Part model, mm, in its own coordinate system. A direction names the side the tool comes from. Give positions to 0.01 mm unless a question says otherwise; leave off trailing zeros. Write each loop counter-clockwise with the first axis right and the second up, starting at its lowest first coordinate (ties: lowest second). Pieces come first, ordered by that corner, then holes. Notation, with made-up numbers: (-12.5, 3) - (17.5, 3) arc R24 cw to (17.5, 34) - close; hole circle Ø9 at (16, 22.5). An arc over 180 degrees is marked (long way). Answer in a Markdown table with one row per item. Add a question column.
1. Probe line 1 along X through (y, z) = (-5.5, 216); line 2 along Z through (x, y) = (-749.3, -17.5); line 3 along Z through (x, y) = (-891.5, -16). List the from-to ranges inside material, lowest first.
2. Band-saw the part on A-A on y = -15.25. State how many separate pieces and enclosed holes the cut face has, plus the area to 3 significant figures.
3. Which spindle directions (+Z, -Z, +X, -X, +Y, -Y) get a long thin tool onto all of the face, cutting with end or side? Do faces 1 (the flat face through (-1172, -13, 152.4)), 2 (the flat face through (-1473.2, -13, 283)), 3 (the flat face through (-1161, -13, 410.362)). Say none if no direction does.
4. Drop flat-ended pins along their axis: pin 1 Ø3 at (x, z) = (-1460.5, 363.93) entering from +Y; pin 2 Ø3 at (x, z) = (-60.5, 475) entering from +Y; pin 3 Ø1 at (x, y) = (-856.5, -18) entering from -Z. Give the stop position or say it passes through.
5. Band-saw the part on B-B on z = 448. Write the cut outline in (x, y).
```python
from build123d import *

# Parameters (mm, degrees)
F1_DEPTH       = 12.7
F3_D           = 4.826
F4_DEPTH       = 25.4
F7_D           = 4.826
F7_ON_F6_D     = 4.826
F9_D           = 4.826
F9_CBORE_D     = 9.4742
F9_CBORE_DEPTH = 5.08


with BuildPart() as f1:
    # F0 (on Front) → F1 (new body)
    with BuildSketch(Plane.XZ):
        with BuildLine():
            Line((-1447.8, 410.3624), (-1473.2, 384.9624))
            Line((-1473.2, 384.9624), (-1473.2, 382.9812))
            Line((-1473.2, 382.9812), (-1422.4, 382.9812))
            Line((-1422.4, 382.9812), (-1422.4, 344.8812))
            Line((-1422.4, 344.8812), (-762, 344.8812))
            Line((-762, 344.8812), (-723.9, 344.8812))
            Line((-723.9, 344.8812), (-711.2, 344.8812))
            Line((-711.2, 344.8812), (-711.2, 217.8812))
            Line((-711.2, 217.8812), (-723.9, 217.8812))
            Line((-723.9, 217.8812), (-762, 217.8812))
            Line((-762, 217.8812), (-1422.4, 217.8812))
            Line((-1422.4, 217.8812), (-1422.4, 179.7812))
            Line((-1422.4, 179.7812), (-1473.2, 179.7812))
            Line((-1473.2, 179.7812), (-1473.2, 177.8))
            Line((-1473.2, 177.8), (-1447.8, 152.4))
            Line((-1447.8, 152.4), (-887.9453407126, 152.4))
            ThreePointArc((-887.9453407126, 152.4), (-804.116072485, 120.8025879546), (-762, 41.7331305265))
            Line((-762, 41.7331305265), (-736.6, 16.3331305265))
            Line((-736.6, 16.3331305265), (-25.4, 16.3331305265))
            Line((-25.4, 16.3331305265), (0, 41.7331305265))
            Line((0, 41.7331305265), (0, 495.6292694735))
            Line((0, 495.6292694735), (-25.4, 521.0292694735))
            Line((-25.4, 521.0292694735), (-736.6, 521.0292694735))
            Line((-736.6, 521.0292694735), (-762, 495.6292694735))
            ThreePointArc((-762, 495.6292694735), (-808.3643419956, 433.8512711856), (-881.9472626468, 410.3624))
            Line((-881.9472626468, 410.3624), (-1447.8, 410.3624))
        make_face()
    extrude(amount=F1_DEPTH)

    # F3 (through all)
    with Locations(Plane.XZ.offset(12.7)):
        with Locations((-457.2, 415.7218), (-152.4, 415.7218), (-152.4, 134.3406), (-457.2, 134.3406)):
            Hole(F3_D / 2)

    # F0 (on Front) → F4 (join)
    with BuildSketch(Plane.XZ):
        with BuildLine():
            Line((-1447.8, 410.3624), (-1473.2, 384.9624))
            Line((-1473.2, 384.9624), (-1473.2, 382.9812))
            Line((-1473.2, 382.9812), (-1422.4, 382.9812))
            Line((-1422.4, 382.9812), (-1422.4, 344.8812))
            Line((-1422.4, 344.8812), (-762, 344.8812))
            Line((-762, 344.8812), (-723.9, 344.8812))
            Line((-723.9, 344.8812), (-711.2, 344.8812))
            Line((-711.2, 344.8812), (-711.2, 217.8812))
            Line((-711.2, 217.8812), (-723.9, 217.8812))
            Line((-723.9, 217.8812), (-762, 217.8812))
            Line((-762, 217.8812), (-1422.4, 217.8812))
            Line((-1422.4, 217.8812), (-1422.4, 179.7812))
            Line((-1422.4, 179.7812), (-1473.2, 179.7812))
            Line((-1473.2, 179.7812), (-1473.2, 177.8))
            Line((-1473.2, 177.8), (-1447.8, 152.4))
            Line((-1447.8, 152.4), (-887.9453407126, 152.4))
            ThreePointArc((-887.9453407126, 152.4), (-804.116072485, 120.8025879546), (-762, 41.7331305265))
            Line((-762, 41.7331305265), (-736.6, 16.3331305265))
            Line((-736.6, 16.3331305265), (-25.4, 16.3331305265))
            Line((-25.4, 16.3331305265), (0, 41.7331305265))
            Line((0, 41.7331305265), (0, 495.6292694735))
            Line((0, 495.6292694735), (-25.4, 521.0292694735))
            Line((-25.4, 521.0292694735), (-736.6, 521.0292694735))
            Line((-736.6, 521.0292694735), (-762, 495.6292694735))
            ThreePointArc((-762, 495.6292694735), (-808.3643419956, 433.8512711856), (-881.9472626468, 410.3624))
            Line((-881.9472626468, 410.3624), (-1447.8, 410.3624))
        make_face()
        Polygon((-1422.4, 382.9812), (-1473.2, 382.9812), (-1473.2, 344.8812), (-1460.5, 344.8812), (-1435.1, 344.8812), (-1422.4, 344.8812), align=None)
        Polygon((-1460.5, 344.8812), (-1473.2, 344.8812), (-1473.2, 281.3812), (-1473.2, 217.8812), (-1460.5, 217.8812), (-1435.1, 217.8812), (-1422.4, 217.8812), (-762, 217.8812), (-723.9, 217.8812), (-711.2, 217.8812), (-711.2, 344.8812), (-723.9, 344.8812), (-762, 344.8812), (-1422.4, 344.8812), (-1435.1, 344.8812), align=None)
        Polygon((-1460.5, 217.8812), (-1473.2, 217.8812), (-1473.2, 179.7812), (-1422.4, 179.7812), (-1422.4, 217.8812), (-1435.1, 217.8812), align=None)
    extrude(amount=F4_DEPTH)

    # F7 (through all)
    with Locations(Plane.XZ.offset(25.4)):
        with Locations((-1460.5, 363.9312), (-1435.1, 363.9312), (-1435.1, 198.8312), (-1460.5, 198.8312), (-749.3, 198.8312), (-723.9, 198.8312), (-749.3, 363.9312), (-723.9, 363.9312)):
            Hole(F7_D / 2)

    # F7 on F6 (through all)
    with Locations(Plane.XZ.offset(25.4)):
        with Locations((-457.2, 345.8718), (-152.4, 345.8718), (-152.4, 216.8906), (-457.2, 216.8906)):
            Hole(F7_ON_F6_D / 2)

    # F9 (through all)
    with Locations(Plane(origin=(0, 0, 0), x_dir=(1, 0, 0), z_dir=(0, 1, 0))):
        with Locations((-34.1376, -63.1199305265), (-59.5122, -63.1199305265), (-34.1376, -20.3463305265), (-59.5122, -20.3463305265), (-59.5122, -517.0160694735), (-34.1376, -517.0160694735), (-34.1376, -474.2424694735), (-59.5122, -474.2424694735)):
            CounterBoreHole(F9_D / 2, F9_CBORE_D / 2, F9_CBORE_DEPTH)


solid = f1.part
```
Values:
| question | item | result |
|---|---|---|
| 1 | line 1 | x = -1473.2 to -459.44, -454.96 to -154.64, -150.16 to 0 |
| 1 | line 2 | z = 29.03 to 196.42, 201.24 to 361.52, 366.34 to 508.33 |
| 1 | line 3 | z = 152.4 to 410.36 |
| 2 | separate pieces | 1 |
| 2 | enclosed holes | 20 |
| 2 | area | 572,000 mm² |
| 3 | face 1 | -Z, -X, +Y, -Y |
| 3 | face 2 | +Z, -Z, -X, +Y, -Y |
| 3 | face 3 | +Z, -X, +Y, -Y |
| 4 | pin 1 | passes through |
| 4 | pin 2 | stops at y = -5.08 |
| 4 | pin 3 | stops at z = 148.32 |
| 5 | outline | (-791.71, -25.4) - (0, -25.4) - (0, 0) - (-791.71, 0) - close |
